```python
from build123d import *

# Parameters (mm, degrees)
BOSS_EXTRUDE1_DEPTH = 12.446
BOSS_EXTRUDE3_DEPTH = 3.175
FILLET1_R           = 1.905
SKETCH7_R           = 3.175
SKETCH8_R           = 3.937
CUT_EXTRUDE3_DEPTH  = 5.08
SKETCH9_R           = 2.5527
CUT_EXTRUDE4_DEPTH  = 47.541246528


with BuildPart() as part:
    # Sketch1 → Boss-Extrude1 (new body)
    with BuildSketch(Plane(origin=(0, 0, 0), x_dir=(0, 0, -1), z_dir=(1, 0, 0))):
        Polygon((0, -28.2575), (15.24, 0), (0, 28.2575), (-15.24, 0), align=None)
    extrude(amount=BOSS_EXTRUDE1_DEPTH)

    # Sketch6 → Boss-Extrude3 (add)
    with BuildSketch(Plane(origin=(12.446, 0, 0), x_dir=(0, 0, -1), z_dir=(1, 0, 0))):
        Polygon((-22.454651823, 0), (0, -41.634666921), (22.454651823, 0), (0, 41.634666921), align=None)
    extrude(amount=BOSS_EXTRUDE3_DEPTH)

    # Fillet1
    fillet1_edges = [part.edges().sort_by_distance(p)[0] for p in [
        (14.0335, 41.634666921, 0),
        (14.0335, 0, 22.454651823),
        (14.0335, -41.634666921, 0),
        (14.0335, 0, -22.454651823),
        (6.223, 0, -15.24),
        (6.223, -28.2575, 0),
        (6.223, 0, 15.24),
        (6.223, 28.2575, 0),
    ]]
    fillet(fillet1_edges, radius=FILLET1_R)

    # Sketch7 → Cut-Revolve2 (revolve, cut)
    with BuildSketch(Plane(origin=(0, 0, 0), x_dir=(1, 0, 0), z_dir=(0, 1, 0))):
        with Locations((6.096, 0)):
            Circle(SKETCH7_R)
    revolve(axis=Axis((15.875, 0, 0), (0, 0, 1)), mode=Mode.SUBTRACT)

    # Sketch8 → Cut-Extrude3 (cut)
    with BuildSketch(Plane(origin=(15.621, 0, 0), x_dir=(0, 0, -1), z_dir=(1, 0, 0))):
        with Locations((8.89, 0)):
            Circle(SKETCH8_R)
        with Locations(Location((-8.89, 0, 0), (0, 0, 180))):
            Circle(SKETCH8_R)
    extrude(amount=-CUT_EXTRUDE3_DEPTH, mode=Mode.SUBTRACT)

    # Sketch9 → Cut-Extrude4 (cut, through all)
    with BuildSketch(Plane(origin=(10.541, 0, 0), x_dir=(0, 0, -1), z_dir=(1, 0, 0))):
        with Locations((8.89, 0)):
            Circle(SKETCH9_R)
        with Locations(Location((-8.89, 0, 0), (0, 0, 180))):
            Circle(SKETCH9_R)
    extrude(amount=-CUT_EXTRUDE4_DEPTH, mode=Mode.SUBTRACT)


solid = part.part
```
Can you work these out from the model? Positions are in its coordinate system, mm. A direction names the side the tool comes from. Give positions to 0.01 mm unless a question says otherwise; leave off trailing zeros. Loops run counter-clockwise (first coordinate to the right, second up) from the corner with the lowest first, then second, coordinate; pieces in that order, holes last. Notation, with made-up numbers: M 60,62 L 77,62 A25 ccw 77,100 Z; hole C 53.25,18 d11. An arc over 180 degrees is marked long. One line per item, written item: value.
(1) Suppose I cut it at C-C on x = 14. Count the separate pieces of the cut face and the enclosed holes in it, plus the area to 3 significant figures.
Returned:
separate pieces: 1
enclosed holes: 4
area: 1,700 mm^2
(2) I need wall thicknesses on line 1 (Y direction, x = 13.5, z = -8.89); line 2 (Z direction, x = 8.25, y = -1.5); line 3 (Z direction, x = 4.75, y = -1). Which ranges of each line are inside material? Lowest first, please.
Returned:
line 1: -25.15 to -3.94, 3.94 to 25.15
line 2: -14.43 to -10.96, -6.82 to -2.46, 2.46 to 6.82, 10.96 to 14.43
line 3: -14.7 to -11.24, -6.54 to -2.85, 2.85 to 6.54, 11.24 to 14.7
(3) Will these pins go through, and if not, where does the flat tip stop? pin 1 (4 mm diameter, centred on x = 5, z = -10, fed in from -Y); pin 2 (3 mm diameter, centred on x = 9.5, y = 18.5, fed in from -Z); pin 3 (4 mm diameter, centred on y = 0, z = -9.5, fed in from +X).
Returned:
pin 1: y = -13.42
pin 2: z = -6.07
pin 3: x = 10.54
(4) Which directions (+Z, -Z, +X, -X, +Y, -Y) give clear straight access to the entire face, cutting with the end or side of a thin tool? Please do faces 5 (the face through (6.31, 0.01, 14.98)), 6 (the face through (6.31, 26.15, -0.03)), 7 (the face through (6.136, -12.857, 8.306)), 8 (the face through (13.12, 2.4, 5.77)).
Returned:
face 5: +Z, -X
face 6: -X, +Y
face 7: +Z, -X, -Y
face 8: +X
(5) We'd pull the mould along Z, two halves only. Please class faces 1 (the face through (10.541, 3, 9)), 2 (the face through (10.541, -3, -9)), 3 (the face through (14.056, 39.526, 0.029)), 4 (the face through (6.136, 12.857, -8.306)): released by +Z, released by -Z, zero draft, split by the parting line, or undercut.
Returned:
face 1: undercut
face 2: undercut
face 3: split by the parting line
face 4: released by -Z
(6) Suppose I cut it at A-A on y = -22. List the corners of the cut face in (x, z) for me, plus the area to 3 significant figures.
Returned:
outline: M 0,-3.37 L 12.45,-3.37 L 12.45,-10.59 L 15.62,-10.59 L 15.62,10.59 L 12.45,10.59 L 12.45,3.37 L 0,3.37 Z
area: 151 mm^2
(7) Suppose I cut it at B-B on z = -8.89. List the corners of the cut face in (x, y) for me, plus the area to 3 significant figures.
Returned:
outline: M 0,-11.77 L 12.45,-11.77 L 12.45,-25.15 L 15.62,-25.15 L 15.62,-3.94 L 10.54,-3.94 L 10.54,-2.55 L 0,-2.55 Z; M 0,2.55 L 10.54,2.55 L 10.54,3.94 L 15.62,3.94 L 15.62,25.15 L 12.45,25.15 L 12.45,11.77 L 0,11.77 Z
area: 359 mm^2
